Autodesk Inventor part; units mm, degrees
ref_plane "YZ Plane" through (0, 0, 0) normal (1, 0, 0) x (0, 1, 0)
ref_plane "XZ Plane" through (0, 0, 0) normal (0, 1, 0) x (-1, 0, 0)
ref_plane "XY Plane" through (0, 0, 0) normal (0, 0, 1) x (1, 0, 0)
sketch "Sketch1" plane through (0, 0, 0) normal (0, 0, 1) x (1, 0, 0)
  line L0 (0, 0) -> (0, 20)
  circle A0 centre (0, 20) radius 1.5
  circle A1 centre (0, 0) radius 1.5
  line L1 (-5, 25) -> (5, 25)
  line L2 (5, 25) -> (5, -5)
  line L3 (5, -5) -> (-5, -5)
  line L4 (-5, -5) -> (-5, 25)
  dimension "d0" = 20
  dimension "d1" = 3
  dimension "d2" = 3
  dimension "d3" = 5
  dimension "d4" = 5
  dimension "d5" = 10
  dimension "d6" = 5
extrude "Extrusion1" add sketch "Sketch1" along normal blind 8
sketch "Sketch2" plane through (5, -5, 0) normal (1, 0, 0) x (0, 0, -1)
  line L0 (-8, 0) -> (-132.5098, -148.385)
  line L1 (-132.5098, -148.385) -> (-124.5098, -148.385)
  line L2 (-124.5098, -148.385) -> (1.3551, 1.615)
  line L3 (-8, 0) -> (-8, 30)
  line L4 (0, 0) -> (0, 30)
  line L5 (0, 30) -> (-8, 30)
  line L6 (-8, 0) -> (-8, 30)
  line L7 (0, 0) -> (-8, 0)
  point P0 (0, 5)
  point P1 (0, 0)
  dimension "d9" = 8
  dimension "d10" = 140
  dimension "d11" = 150
extrude "Extrusion2" add sketch "Sketch2" against normal up to surface (10 mm away) contours L7 L2 L1 L0
chamfer "Chamfer1" distance 2 angle 45 2 edges at (-1.5, 20, 8) (-1.5, 0, 8)
fillet "Fillet1" radius 4 2 edges at (5, 25, 4) (-5, 25, 4)
sketch "Sketch3" plane through (5, -153.385, 132.5098) normal (1, 0, 0) x (0, 0, -1)
  line L0 (0, 0) -> (8, 0)
  line L1 (8, 0) -> (132.5098, 0)
  line L2 (132.5098, 0) -> (132.5098, 5)
  line L3 (132.5098, 5) -> (8, 5)
  line L4 (8, 5) -> (8, 0)
  line L5 (132.5098, 148.6932) -> (124.5098, 148.6932)
  line L6 (124.5098, 148.6932) -> (124.5098, 0)
  line L7 (124.5098, 0) -> (132.5098, 0)
  line L8 (132.5098, 0) -> (132.5098, 148.6932)
  line L9 (124.5098, 148.385) -> (124.5098, 174.385)
  line L10 (124.5098, 148.385) -> (0, 0)
  line L11 (75.519, 90) -> (80.519, 90)
  line L12 (80.519, 90) -> (80.519, 0)
  line L13 (80.519, 0) -> (75.519, 0)
  line L14 (75.519, 0) -> (75.519, 90)
  line L15 (8, 0) -> (132.5098, 148.385)
  line L16 (132.5098, 65) -> (58.346, 65)
  line L17 (58.346, 65) -> (58.346, 60)
  line L18 (58.346, 60) -> (132.5098, 60)
  line L19 (132.5098, 60) -> (132.5098, 65)
  point P0 (132.5098, 153.385)
  point P1 (132.5098, 5)
  point P2 (124.5098, 5)
  point P3 (80.519, 5)
  point P4 (75.519, 5)
  point P5 (80.519, 60)
  point P6 (124.5098, 60)
  point P7 (124.5098, 65)
  point P8 (80.519, 65)
  point P9 (75.519, 60)
  point P10 (75.519, 65)
  dimension "d18" = 5
  dimension "d19" = 5
  dimension "d20" = 90
  dimension "d23" = 5
  dimension "d24" = 55
extrude "Extrusion3" add sketch "Sketch3" against normal blind 10 contours L15 L3 L14 L1 | L4 L3 L15 | L11 L12 L15 L14 | L14 L3 L12 L1 | L6 L5 L8 L15 | L15 L12 L16 L14 | L12 L3 L6 L1 | L14 L18 L12 L3 | L17 L16 L15 | L15 L16 L14 L18 | L15 L8 L16 L6 | L16 L12 L18 L14 | L6 L3 L2 L1 | L16 L8 L18 L6 | L6 L18 L12 L16 | L6 L18 L8 L3
properties part number "legs"
Check sheet for the modelled part. Datum: model origin and axes. Units: mm. A direction names the side the tool comes from. Coordinates: 2 decimals unless noted, no trailing zeros. Loops run counter-clockwise (first coordinate to the right, second up) from the corner with the lowest first, then second, coordinate; pieces in that order, holes last. Notation, with made-up numbers: (35, 8) -> (68, 8) arc R8 cw to (68, 20) -> close; hole circle Ø1 at (-32.5, -20.75). An arc over 180 degrees is marked (long way). Write item = value, one per line. Start each with the question number.
1. Tool access check on faces 1 (the flat face through (0, -153.385, 67)), 2 (the flat face through (0, -120, 8)), 3 (the flat face through (0, 10, 8)). Record the directions out of +Z, -Z, +X, -X, +Y, -Y that give a thin tool (end or side, any length) a straight path to the whole face; none if there is none.
2. Depth check by flat-ended pin: P1, Ø3, axis at x = 0, z = 21.5, coming from the +Y side; P2, Ø3, axis at x = 0.5, y = -64.5, coming from the +Z side; P3, Ø3, axis at x = 1, z = 66.5, coming from the +Y side. Enter the tip coordinate at first touch or a pass-through.
3. Section check B-B on z = 39. Record the cut outline in (x, y) (3 decimals), then the cut area to 3 significant figures.
4. Section check C-C on y = -44. Record the cut outline in (x, z), then the cut area to 3 significant figures.
5. Section check A-A on y = -128.5. Record the cut outline in (x, z), then the cut area to 3 significant figures.
6. Draft check along Z on faces 4 (the flat face through (0, -63, 0)), 5 (the conical face through (0.874, 21.37, 6.125)), 6 (the flat face through (0.07, -121.27, 97.56)). Enter one of: released by +Z, released by -Z, zero draft, split by the parting line, or undercut.
7. Material ranges on line 1 (Y direction, x = 0, z = 2.4) (3 decimals); line 2 (X direction, y = 20, z = 2); line 3 (Z direction, x = -3.75, y = -85), recorded low to high.
Responses:
q1.face_1 = +Z, -Z, +X, -X, -Y
q1.face_2 = +X, -X
q1.face_3 = +Z, +X, -X, +Y
q2.P1 = -19.3
q2.P2 = 59.19
q2.P3 = -72.93
q3.outline = (-5, -153.385) -> (5, -153.385) -> (5, -148.385) -> (-5, -148.385) -> close; (-5, -93.385) -> (5, -93.385) -> (5, -88.385) -> (-5, -88.385) -> close; (-5, -51.478) -> (5, -51.478) -> (5, -41.944) -> (-5, -41.944) -> close
q3.area = 195 mm2
q4.outline = (-5, 0) -> (5, 0) -> (5, 8) -> (-5, 8) -> close; (-5, 32.72) -> (5, 32.72) -> (5, 40.72) -> (-5, 40.72) -> close
q4.area = 160 mm2
q5.outline = (-5, 0) -> (5, 0) -> (5, 8) -> (-5, 8) -> close; (-5, 51.99) -> (5, 51.99) -> (5, 56.99) -> (-5, 56.99) -> close; (-5, 103.63) -> (5, 103.63) -> (5, 111.63) -> (-5, 111.63) -> close
q5.area = 210 mm2
q6.face_4 = released by -Z
q6.face_5 = released by +Z
q6.face_6 = undercut
q7.line_1 = -153.385 to -1.5, 1.5 to 18.5, 21.5 to 25
q7.line_2 = -5 to -1.5, 1.5 to 5
q7.line_3 = 0 to 8, 51.99 to 56.99, 67.13 to 75.13
